Check sheet for the drawn part. Datum: minimum x, y, z corner. Units: mm. A direction names the side the tool comes from. Round coordinates to 2 decimals unless told otherwise and drop trailing zeros. Write each loop counter-clockwise with the first axis right and the second up, starting at its lowest first coordinate (ties: lowest second). Pieces come first, ordered by that corner, then holes. Notation, with made-up numbers: (-5.75, 68.5) -> (15.25, 68.5) arc R20 cw to (15.25, 79.5) -> close; hole circle Ø4 at (-37, -1.75). An arc over 180 degrees is marked (long way). Use a Markdown table: item, result.
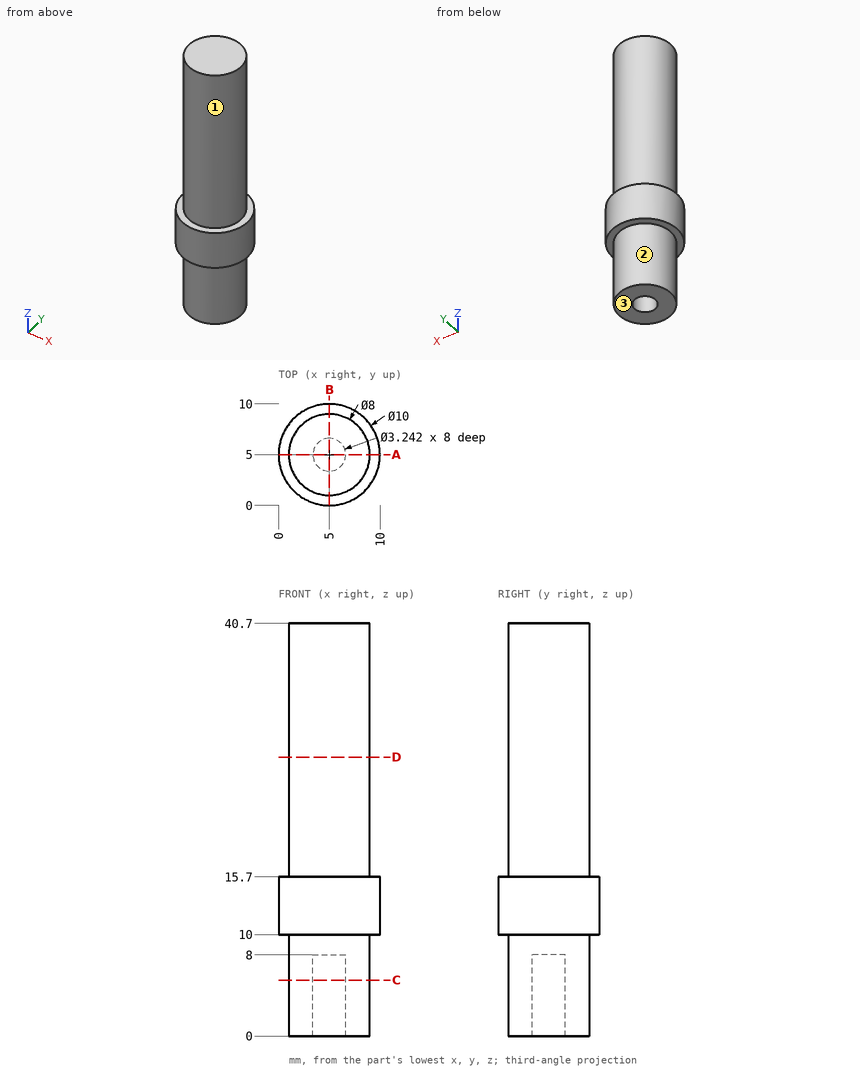
(1) Thickness scan on line 1 (Y direction, x = 5, z = 5.25); line 2 (Y direction, x = 5.25, z = 19); line 3 (Y direction, x = 4.5, z = 4). Record the ranges inside material, lowest first.
A:
| item | result |
|---|---|
| line 1 | y = 1 to 3.38, 6.62 to 9 |
| line 2 | y = 1.01 to 8.99 |
| line 3 | y = 1.03 to 3.46, 6.54 to 8.97 |
(2) Section check D-D on z = 27.5. Record the cut outline in (x, y), plus the area to 3 significant figures.
A:
| item | result |
|---|---|
| outline | circle Ø8 at (5, 5) |
| area | 50.3 mm2 |
(3) Section check C-C on z = 5.5. Record the cut outline in (x, y), plus the area to 3 significant figures.
A:
| item | result |
|---|---|
| outline | circle Ø8 at (5, 5); hole circle Ø3.24 at (5, 5) |
| area | 42.0 mm2 |
(4) Access from +Z, -Z, +X, -X, +Y, -Y to the whole of each face (thin tool, end or side, straight path). Record for the marked faces 1, 2 and 3.
A:
| item | result |
|---|---|
| face 1 | +Z |
| face 2 | -Z |
| face 3 | -Z, +X, -X, +Y, -Y |
(5) Section check A-A on y = 5. Record the cut outline in (x, z), plus the area to 3 significant figures.
A:
| item | result |
|---|---|
| outline | (0, 10) -> (1, 10) -> (1, 0) -> (3.38, 0) -> (3.38, 8) -> (6.62, 8) -> (6.62, 0) -> (9, 0) -> (9, 10) -> (10, 10) -> (10, 15.7) -> (9, 15.7) -> (9, 40.7) -> (1, 40.7) -> (1, 15.7) -> (0, 15.7) -> close |
| area | 311 mm2 |
(6) Gauge pin test, flat ends, axial feed: pin 1 Ø5 at (x, y) = (3, 3) entering from -Z; pin 2 Ø1.5 at (x, z) = (6, 7.5) entering from -Y; pin 3 Ø2 at (y, z) = (7.5, 8) entering from +X; pin 4 Ø1 at (x, y) = (5.5, 4.5) entering from -Z. Record the tip position at first contact, or that the pin passes through.
A:
| item | result |
|---|---|
| pin 1 | stops at z = 0 |
| pin 2 | stops at y = 1.01 |
| pin 3 | stops at x = 8.71 |
| pin 4 | stops at z = 8 |
